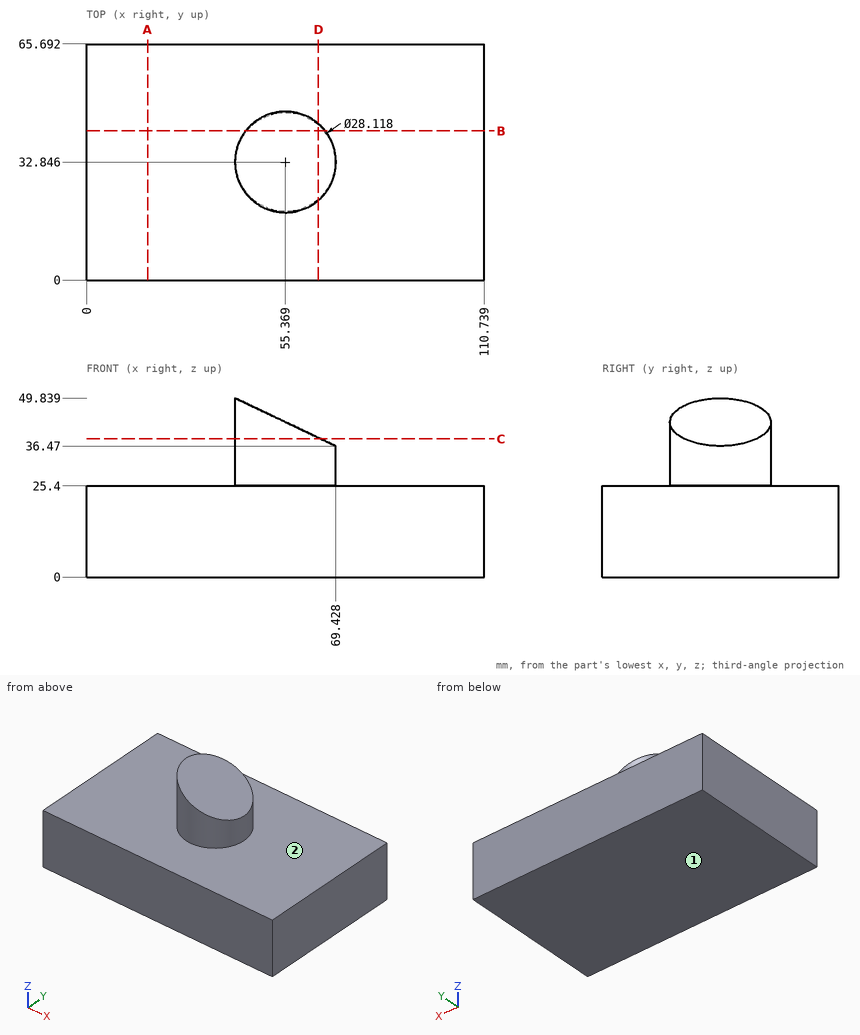
Design review of the part shown in the three views and the two pictorial views. Dimensions are in mm from the part's minimum x, y and z. A direction names the side the tool comes from. Round coordinates to 2 decimals unless told otherwise and drop trailing zeros. Loops run counter-clockwise (first coordinate to the right, second up) from the corner with the lowest first, then second, coordinate; pieces in that order, holes last.
1) Consider section C-C on z = 38.5. State the section outline as (x, y) points (1 decimal).
Values follow:
outline: (65.2, 22.8) - (65.2, 42.9) arc R14.1 ccw (long way) to start
2) Tool access review of the marked faces 1 and 2: name each direction out of +Z, -Z, +X, -X, +Y, -Y from which nothing blocks a thin tool from reaching the whole face with its end or side.
Values follow:
face 1: -Z, +X, -X, +Y, -Y
face 2: +Z
3) Wall thickness on line 1 along Z through (x, y) = (84.5, 62.5); line 2 along Z through (x, y) = (63, 25) (1 decimal); line 3 along X through (y, z) = (20, 28.5) (1 decimal): over which ranges is each line inside the solid? List them lowest first.
Values follow:
line 1: z = 0 to 25.4
line 2: z = 0 to 39.5
line 3: x = 49.7 to 61.1
4) Consider section D-D on x = 64.5. State the section outline as (y, z) points (1 decimal).
Values follow:
outline: (0, 0) - (65.7, 0) - (65.7, 25.4) - (43.5, 25.4) - (43.5, 38.8) - (22.2, 38.8) - (22.2, 25.4) - (0, 25.4) - close
5) Consider section A-A on x = 17. State the section outline as (y, z) points, then the cut area to 3 significant figures.
Values follow:
outline: (0, 0) - (65.69, 0) - (65.69, 25.4) - (0, 25.4) - close
area: 1,670 mm2
6) Clearance check with a flat-ended pin moving along its axis: P1, Ø10, axis at x = 38, y = 57, coming from the +Z side. State where the tip first meets the part, or that it passes through.
Values follow:
P1: stops at z = 25.4
7) Consider section B-B on y = 41.5. State the section outline as (x, z) points, then the cut area to 3 significant figures.
Values follow:
outline: (0, 0) - (110.74, 0) - (110.74, 25.4) - (66.45, 25.4) - (66.45, 37.89) - (44.29, 48.42) - (44.29, 25.4) - (0, 25.4) - close
area: 3,210 mm2
